Could you check a few things on this model? Use its own coordinates, in mm. Face numbers are marked on the shaded views. A direction names the side the tool comes from. Give positions to 0.01 mm unless a question says otherwise; leave off trailing zeros. Write each loop counter-clockwise with the first axis right and the second up, starting at its lowest first coordinate (ties: lowest second). Pieces come first, ordered by that corner, then holes. Notation, with made-up numbers: M 81,-12.75 L 115,-12.75 A17 cw 115,3.25 Z; hole C 85,41.25 d2. An arc over 180 degrees is marked long. Use one line per item in the form item = value.
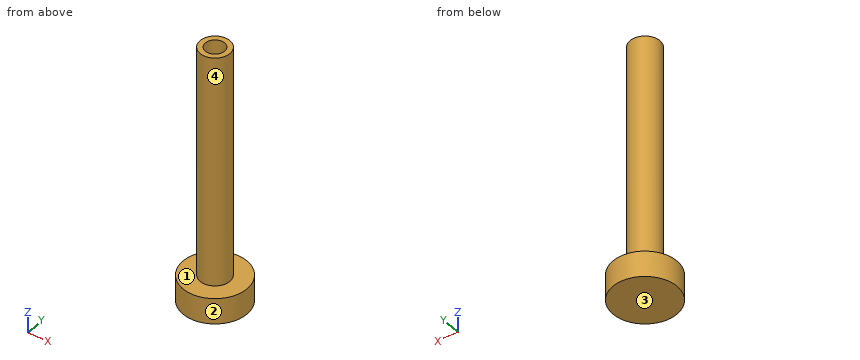
from build123d import *

# Parameters (mm, degrees)
F0_R     = 2.325
F1_DEPTH = 40
F0_R_2   = 5
F2_DEPTH = 4
F3_R     = 1.5
F4_DEPTH = 12


with BuildPart() as f1:
    # F0 (on Top) → F1 (new body)
    with BuildSketch(Plane.XY):
        Circle(F0_R)
    extrude(amount=F1_DEPTH)

    # F0 (on Top) → F2 (join)
    with BuildSketch(Plane.XY):
        Circle(F0_R_2)
        Circle(F0_R, mode=Mode.SUBTRACT)
    extrude(amount=F2_DEPTH)

    # F3 (on face) → F4 (cut)
    with BuildSketch(Plane.XY.offset(40)):
        Circle(F3_R)
    extrude(amount=-F4_DEPTH, mode=Mode.SUBTRACT)


solid = f1.part
1) Thinking about a two-plate mould opening in Y: for the marked faces 3 and 4, which applies, released by +Y, released by -Y, zero draft, split by the parting line, or undercut?
Checked values:
face_3 = zero draft
face_4 = split by the parting line
2) I want a section at C-C, the plane z = 37. Please give me the cut outline in (x, y) (3 decimals).
Checked values:
outline = C 0,0 d4.65; hole C 0,0 d3
3) I want a section at D-D, the plane z = 6.5. Please give me the cut outline in (x, y) (3 decimals), plus the area to 3 significant figures.
Checked values:
outline = C 0,0 d4.65
area = 17.0 mm2
4) For pin 1 Ø6 at (x, y) = (-1, -3) entering from +Z; pin 2 Ø2 at (y, z) = (2.5, 15.5) entering from +X; pin 3 Ø2 at (y, z) = (0, 20) entering from +X (3 decimals); pin 4 Ø3 at (x, z) = (1.5, 16) entering from -Y (3 decimals), each with a flat end and sliding along its axis, tell me the tip position at first contact or that it passes through.
Checked values:
pin_1 = 40
pin_2 = 1.78
pin_3 = 2.325
pin_4 = -2.325
5) I want a section at A-A, the plane x = 0. Please give me the cut outline in (y, z) (3 decimals).
Checked values:
outline = M -5,0 L 5,0 L 5,4 L 2.325,4 L 2.325,40 L 1.5,40 L 1.5,28 L -1.5,28 L -1.5,40 L -2.325,40 L -2.325,4 L -5,4 Z
6) For the marked faces 1 and 2, which set-ups out of +Z, -Z, +X, -X, +Y, -Y let a thin tool reach every point of the face, with its end or its side?
Checked values:
face_1 = +Z
face_2 = +Z, -Z
7) If I drill on L1, parallel to Y at x = 0, z = 32 (3 decimals); L2, parallel to Z at x = -4.5, y = -1.75; L3, parallel to Z at x = -0.75, y = 0.25, over which ranges is the centre line in solid material (lowest first)?
Checked values:
L1 = -2.325 to -1.5, 1.5 to 2.325
L2 = 0 to 4
L3 = 0 to 28
